Read the model definition and answer for the solid it produces. Units are mm, in the model's axes. Face numbers are marked on the shaded views. A direction names the side the tool comes from. Round coordinates to 2 decimals unless told otherwise and drop trailing zeros. Loops run counter-clockwise (first coordinate to the right, second up) from the corner with the lowest first, then second, coordinate; pieces in that order, holes last. Notation, with made-up numbers: (32.25, -27.5) - (83.25, -27.5) arc R17 cw to (83.25, -4.5) - close; hole circle Ø7 at (65, 35). An arc over 180 degrees is marked (long way). Answer as CSV lines item,"result".
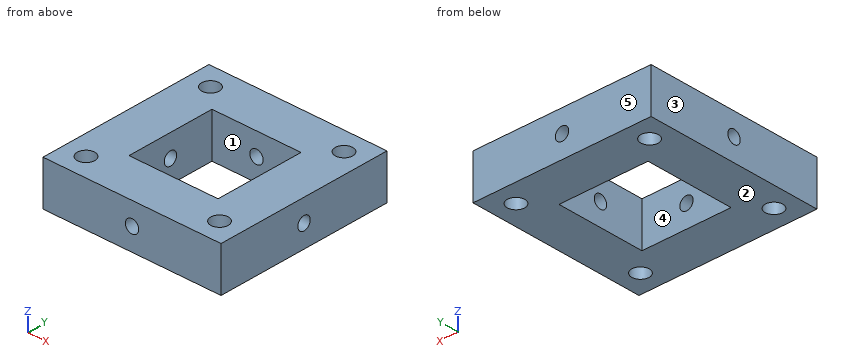
```python
from build123d import *

# Parameters (mm, degrees)
F0_W          = 50.8
F0_H          = 50.8
F1_DEPTH      = 6.35
F1_DEPTH_BACK = 6.35
F2_W          = 25.4
F2_H          = 25.4
F3_DEPTH      = 113.7438993901
F4_D          = 4.9784
F7_D          = 3.7973
F7_ON_F5_D    = 3.7973


with BuildPart() as f1:
    # F0 (on Top) → F1 (new body, two sides)
    with BuildSketch(Plane.XY) as f1_sk:
        with Locations((25.4, 25.4)):
            Rectangle(F0_W, F0_H)
    extrude(amount=F1_DEPTH)
    extrude(f1_sk.sketch, amount=-F1_DEPTH_BACK)

    # F2 (on face) → F3 (cut)
    with BuildSketch(Plane.XY.offset(6.35)):
        with Locations((25.4, 25.4)):
            Rectangle(F2_W, F2_H)
    extrude(amount=-F3_DEPTH, mode=Mode.SUBTRACT)

    # F4 (through all)
    with Locations(Plane.XY.offset(6.35)):
        with Locations((44.45, 44.45), (6.35, 44.45), (6.35, 6.35), (44.45, 6.35)):
            Hole(F4_D / 2)

    # F7 (through all)
    with Locations(Plane.XZ):
        with Locations((25.4, 0)):
            Hole(F7_D / 2)

    # F7 on F5 (through all)
    with Locations(Plane(origin=(0, 0, 0), x_dir=(0, -1, 0), z_dir=(-1, 0, 0))):
        with Locations((-25.4, 0)):
            Hole(F7_ON_F5_D / 2)


solid = f1.part
```
1) A tool of negligible diameter and unlimited length cuts with its end or side. For the marked faces 4 and 5, from which of +Z, -Z, +X, -X, +Y, -Y can it reach the whole face along a straight path? Write none if from no direction.
Entries:
face 4,"+Z, -Z"
face 5,"+Z, -Z, +X, -X, +Y"
2) A cutting plane is placed at D-D, the plane y = 16. Determine the outline of the cut face in (x, z), plus the area to 3 significant figures.
Entries:
outline,"(0, -6.35) - (12.7, -6.35) - (12.7, 6.35) - (0, 6.35) - close; (38.1, -6.35) - (50.8, -6.35) - (50.8, 6.35) - (38.1, 6.35) - close"
area,"323 mm^2"
3) Find the intervals of material crossed by line 1 (Y direction, x = 6.5, z = -2.75); line 2 (Y direction, x = 32.5, z = -1.75), in increasing order.
Entries:
line 1,"y = 0 to 3.87, 8.83 to 41.97, 46.93 to 50.8"
line 2,"y = 0 to 12.7, 38.1 to 50.8"
4) Each of these flat-tipped pins is pushed along its axis until it touches: P1, Ø6, axis at x = 25.4, z = 0, coming from the -Y side; P2, Ø4.5, axis at x = 6.35, y = 44.45, coming from the +Z side. Where does it stop, or does it pass through?
Entries:
P1,"stops at y = 0"
P2,"passes through"
5) The mould has two halves that part along X. Classify the marked faces 1, 2 and 3: pulls with the +X half, pulls with the -X half, needs draft (parallel to the pull), parting line crosses it, or undercut.
Entries:
face 1,"undercut"
face 2,"needs draft"
face 3,"pulls with the -X half"
6) A cutting plane is placed at B-B, the plane z = 0. Determine the outline of the cut face in (x, y), plus the area to 3 significant figures.
Entries:
outline,"(0, 0) - (23.5, 0) - (23.5, 12.7) - (12.7, 12.7) - (12.7, 23.5) - (0, 23.5) - close; (0, 27.3) - (12.7, 27.3) - (12.7, 38.1) - (23.5, 38.1) - (23.5, 50.8) - (0, 50.8) - close; (27.3, 0) - (50.8, 0) - (50.8, 23.5) - (38.1, 23.5) - (38.1, 12.7) - (27.3, 12.7) - close; (27.3, 38.1) - (38.1, 38.1) - (38.1, 27.3) - (50.8, 27.3) - (50.8, 50.8) - (27.3, 50.8) - close; hole circle Ø4.98 at (6.35, 6.35); hole circle Ø4.98 at (6.35, 44.45); hole circle Ø4.98 at (44.45, 6.35); hole circle Ø4.98 at (44.45, 44.45)"
area,"1,660 mm^2"
7) A cutting plane is placed at A-A, the plane y = 6.35. Determine the outline of the cut face in (x, z).
Entries:
outline,"(0, -6.35) - (3.86, -6.35) - (3.86, 6.35) - (0, 6.35) - close; (8.84, -6.35) - (41.96, -6.35) - (41.96, 6.35) - (8.84, 6.35) - close; (46.94, -6.35) - (50.8, -6.35) - (50.8, 6.35) - (46.94, 6.35) - close; hole circle Ø3.8 at (25.4, 0)"
8) A cutting plane is placed at C-C, the plane x = 25.4. Determine the outline of the cut face in (y, z).
Entries:
outline,"(0, -6.35) - (12.7, -6.35) - (12.7, -1.9) - (0, -1.9) - close; (0, 1.9) - (12.7, 1.9) - (12.7, 6.35) - (0, 6.35) - close; (38.1, -6.35) - (50.8, -6.35) - (50.8, -1.9) - (38.1, -1.9) - close; (38.1, 1.9) - (50.8, 1.9) - (50.8, 6.35) - (38.1, 6.35) - close"
